Autodesk Inventor part; units mm, degrees
ref_plane "YZ Plane" through (0, 0, 0) normal (1, 0, 0) x (0, 1, 0)
ref_plane "XZ Plane" through (0, 0, 0) normal (0, 1, 0) x (-1, 0, 0)
ref_plane "XY Plane" through (0, 0, 0) normal (0, 0, 1) x (1, 0, 0)
sketch "Sketch1" plane through (0, 0, 0) normal (0, 1, 0) x (-1, 0, 0)
  line L0 (-48.5, -79) -> (48.5, -79)
  line L1 (48.5, -79) -> (48.5, 79)
  line L2 (48.5, 79) -> (-48.5, 79)
  line L3 (-48.5, 79) -> (-48.5, -79)
  line L4 (-48.5, -79) -> (48.5, 79) construction
  line L5 (48.5, -79) -> (-48.5, 79) construction
  point P0 (0, 0)
  dimension "d0" = 97
  dimension "d1" = 158
extrude "Extrusion1" add sketch "Sketch1" along normal blind 5
sketch "Sketch2" plane through (0, 5, 0) normal (0, 1, 0) x (1, 0, 0)
  circle A0 centre (-41, 76.75) radius 1.75
  line L0 (-48.5, -79) -> (48.5, -79)
  line L1 (48.5, -79) -> (48.5, 79)
  circle A1 centre (43.5, -74.5) radius 1.75
  point P0 (0, 0)
  dimension "d4" = 3.5
  dimension "d5" = 155.75
  dimension "d6" = 89.5
  dimension "d7" = 3.5
  dimension "d8" = 4.5
  dimension "d9" = 5
extrude "Extrusion2" cut sketch "Sketch2" against normal blind 5
sketch "Sketch3" plane through (0, 5, 0) normal (0, 1, 0) x (1, 0, 0)
  line L0 (48.5, -79) -> (48.5, 79)
  line L1 (-48.5, 79) -> (-48.5, -79)
  line L2 (48.5, 73) -> (-48.5, 73)
  line L3 (-48.5, 73) -> (-48.5, -59)
  line L4 (-48.5, -59) -> (48.5, -59)
  line L5 (48.5, -59) -> (48.5, 73)
  line L6 (48.5, 79) -> (-48.5, 79)
  line L7 (-48.5, -79) -> (48.5, -79)
  point P0 (0, 0)
  dimension "d12" = 6
  dimension "d13" = 20
extrude "Extrusion3" add sketch "Sketch3" along normal blind 33 contours L4 L1 L2 L0
sketch "Sketch4" plane through (-48.5, 5, 59) normal (0, 0, 1) x (1, 0, 0)
  line L0 (0, 33) -> (97, 33)
  line L1 (97, 0) -> (0, 0)
  line L2 (97, 33) -> (95, 33)
  line L3 (95, 33) -> (95, 0)
  line L4 (95, 0) -> (97, 0)
  line L5 (97, 0) -> (97, 33)
  point P0 (48.5, -5)
  dimension "d16" = 2
extrude "Extrusion4" add sketch "Sketch4" along normal blind 20
sketch "Sketch5" plane through (0, 5, 0) normal (0, 1, 0) x (1, 0, 0)
  line L0 (31.5, -59) -> (-38.5, -59)
  line L1 (-38.5, -59) -> (-38.5, -72)
  line L2 (-38.5, -72) -> (31.5, -72)
  line L3 (31.5, -72) -> (31.5, -59)
  line L4 (-48.5, -59) -> (-48.5, -79)
  line L5 (46.5, -59) -> (-48.5, -59)
  line L6 (-48.5, -79) -> (46.5, -79)
  point P0 (0, 0)
  dimension "d19" = 70
  dimension "d20" = 10
  dimension "d21" = 7
extrude "Extrusion5" add sketch "Sketch5" along normal blind 15
sketch "Sketch6" plane through (0, 0, 0) normal (0, -1, 0) x (1, 0, 0)
  circle A0 centre (41, 53.6) radius 1.6
  circle A1 centre (17, 56.5) radius 1.6
  circle A2 centre (-12.5, 57.6) radius 1.6
  circle A3 centre (41, -66.4) radius 1.6
  circle A4 centre (-12.5, -66.4) radius 1.6
  line L0 (48.5, 79) -> (48.5, -79)
  line L1 (-48.5, 79) -> (48.5, 79)
  circle A5 centre (17, -21.5) radius 1.6
  point P0 (0, 0)
  dimension "d24" = 3.2
  dimension "d25" = 3.2
  dimension "d26" = 3.2
  dimension "d27" = 3.2
  dimension "d28" = 3.2
  dimension "d29" = 7.5
  dimension "d30" = 25.4
  dimension "d31" = 22.5
  dimension "d32" = 31.5
  dimension "d33" = 61
  dimension "d34" = 21.4
  dimension "d35" = 120
  dimension "d36" = 3.2
  dimension "d37" = 78
extrude "Extrusion6" cut sketch "Sketch6" against normal blind 2
properties part number "source"
For this review, take the finished solid that the model builds, in its own axes (mm). A direction names the side the tool comes from. Give positions to 0.01 mm unless a question says otherwise; leave off trailing zeros. Order: outer loops, then holes, each group sorted by start corner. A loop starts at its lowest first (then second) coordinate and runs counter-clockwise, first axis right, second up. Notation, with made-up numbers: M 79.25,10.5 L 128.25,10.5 A12 ccw 128.25,21.5 Z; hole C 56.25,-14 d10. An arc over 180 degrees is marked long. Answer in a Markdown table with one row per item. Add a question column.
(1) Consider section C-C on y = 13.5. State the section outline as (x, z) points.
(2) For pin 1 (6 mm diameter, centred on x = 11.5, z = 68.5, fed in from +Y); pin 2 (3 mm diameter, centred on x = -41, z = -76.75, fed in from +Y); pin 3 (3 mm diameter, centred on x = -1, z = -75, fed in from +Y); pin 4 (1 mm diameter, centred on x = 41, z = 54, fed in from -Y), all flat-tipped, find the tip position at first contact; note any pin that passes through.
(3) Wall thickness on probe 1 along Z at (x, y) = (41, 0.5); probe 2 along X at (y, z) = (1, 57); probe 3 along Z at (x, y) = (-29.5, 14.5): over which ranges is each line inside the solid? List them lowest first. Write a range as [from, to].
(4) Consider section B-B on x = -12.5. State the section outline as (y, z) points.
(5) Consider section A-A on z = -76.75. State the section outline as (x, y) points.
(6) Mouldability with a two-part tool opening along Z and no side actions: class faces 5 (the face through (41.74, 0.99, 52.18)), 6 (the face through (1, 21, -73)), 7 (the face through (46.5, 22, 69)) as +Z half, -Z half, draft (parallel to the pull), parting line (faces both ways), or undercut.
(7) Consider section D-D on z = 74.5. State the section outline as (x, y) points.
(8) For faces 1 (the face through (31.5, 12, 66)), 2 (the face through (41, 2, 54)), 3 (the face through (48.5, 19, -1)), 4 (the face through (-4, 20, 65)), list the 3-axis set-ups (+Z, -Z, +X, -X, +Y, -Y) from which the entire face can be reached by the end or side of a thin tool; tool diameter is ignored.
Evaluation:
| question | item | result |
|---|---|---|
| 1 | outline | M -48.5,-73 L 48.5,-73 L 48.5,79 L 46.5,79 L 46.5,59 L 31.5,59 L 31.5,72 L -38.5,72 L -38.5,59 L -48.5,59 Z |
| 2 | pin 1 | stops at y = 20 |
| 2 | pin 2 | passes through |
| 2 | pin 3 | stops at y = 5 |
| 2 | pin 4 | stops at y = 2 |
| 3 | probe 1 | z = [-79, -68], [-64.8, 52], [55.2, 79] |
| 3 | probe 2 | x = [-48.5, -13.98], [-11.02, 15.48], [18.52, 48.5] |
| 3 | probe 3 | z = [-73, 72] |
| 4 | outline | M 0,-79 L 5,-79 L 5,-73 L 38,-73 L 38,59 L 20,59 L 20,72 L 5,72 L 5,79 L 0,79 L 0,59.2 L 2,59.2 L 2,56 L 0,56 L 0,-64.8 L 2,-64.8 L 2,-68 L 0,-68 Z |
| 5 | outline | M -48.5,0 L -42.75,0 L -42.75,5 L -48.5,5 Z; M -39.25,0 L 48.5,0 L 48.5,5 L -39.25,5 Z |
| 6 | face 5 | undercut |
| 6 | face 6 | -Z half |
| 6 | face 7 | draft |
| 7 | outline | M -48.5,0 L 41.75,0 L 41.75,5 L -48.5,5 Z; M 45.25,0 L 48.5,0 L 48.5,38 L 46.5,38 L 46.5,5 L 45.25,5 Z |
| 8 | face 1 | +Z, +Y |
| 8 | face 2 | -Y |
| 8 | face 3 | +Z, -Z, +X, +Y, -Y |
| 8 | face 4 | +Z, -X, +Y |
